Work out the finished part from the listing and answer in its coordinate system (mm). Face numbers are marked on the shaded views. Coordinates: 2 decimals unless noted, no trailing zeros. Loops run counter-clockwise (first coordinate to the right, second up) from the corner with the lowest first, then second, coordinate; pieces in that order, holes last. Notation, with made-up numbers: (53, -29) - (94, -29) arc R36 ccw to (94, 6) - close; hole circle Ø7 at (89, 2.5). An arc over 180 degrees is marked (long way). Write each question's results on one line, items separated by ' | '. Start each with the question number.
Item 1: For a pull along X with two mould halves and no side action, classify the marked faces 1 and 2 as +X half, -X half, draft (parallel to the pull), parting line (faces both ways), or undercut.
Item 2: Section B-B, the plane z = -7 is taken. Write down the section's boundary in (x, y).
Item 3: Section A-A, the plane x = -4 is taken. Write down the section's boundary in (y, z).
Item 4: Section D-D, the plane y = 4.5 is taken. Count the separate pieces of the cut face and the enclosed holes in it, plus the area to 3 significant figures.
Item 5: Section C-C, the plane z = 32.06 is taken. Write down the section's boundary in (x, y) (3 decimals), plus the area to 3 significant figures.
Item 6: Consider probe 1 along X at (y, z) = (5.15, -35) (3 decimals); probe 2 along X at (y, z) = (2.3, -21.4) (3 decimals); probe 3 along Z at (x, y) = (17.5, 5). Determine where each line is inside the solid, lowest interval first. Write a range as [from, to].
Item 7: Each of these flat-tipped pins is pushed along its axis until it touches: pin 1 Ø1 at (y, z) = (1, -3) entering from +X; pin 2 Ø10 at (x, z) = (-19.75, 32.06) entering from -Y; pin 3 Ø1.8 at (x, z) = (22.5, -6) entering from +Y; pin 4 Ø3 at (x, z) = (-19.5, 31) entering from +Y. Where does it stop, or does it pass through?
from build123d import *

# Parameters (mm, degrees)
SKETCH1_W           = 50.8
SKETCH1_H           = 50.8
SKETCH1_R           = 1.375
SKETCH1_W_2         = 40.8
SKETCH1_H_2         = 40.8
BOSS_EXTRUDE1_DEPTH = 1.5
SKETCH2_W           = 50.8
SKETCH2_H           = 50.8
SKETCH2_W_2         = 47.8
SKETCH2_H_2         = 47.8
BOSS_EXTRUDE2_DEPTH = 5
FILLET2_R           = 3
BOSS_EXTRUDE3_REACH = 38.504
SKETCH5_R           = 5
SKETCH5_R_2         = 1.375
SKETCH6_R           = 2.55
CUT_EXTRUDE1_DEPTH  = 3
SKETCH7_R           = 1.55
BOSS_EXTRUDE4_DEPTH = 6.5
SKETCH8_R           = 3.125
CUT_EXTRUDE2_DEPTH  = 4
FILLET3_R           = 5
BOSS_EXTRUDE5_DEPTH = 6.5
SKETCH10_R          = 3.125
CUT_EXTRUDE3_DEPTH  = 4
SKETCH11_R          = 1.55
CUT_EXTRUDE4_DEPTH  = 50.27727671
FILLET4_R           = 3


with BuildPart() as part:
    # Sketch1 → Boss-Extrude1 (new body)
    with BuildSketch(Plane(origin=(0, 0, 0), x_dir=(1, 0, 0), z_dir=(0, 1, 0))):
        Rectangle(SKETCH1_W, SKETCH1_H)
        with Locations(Location((-21.4, 21.4, 0), (0, 0, 270))):
            Circle(SKETCH1_R, mode=Mode.SUBTRACT)
        with Locations(Location((21.4, 21.4, 0), (0, 0, 270))):
            Circle(SKETCH1_R, mode=Mode.SUBTRACT)
        with Locations(Location((21.4, -21.4, 0), (0, 0, 270))):
            Circle(SKETCH1_R, mode=Mode.SUBTRACT)
        with Locations(Location((-21.4, -21.4, 0), (0, 0, 270))):
            Circle(SKETCH1_R, mode=Mode.SUBTRACT)
        Rectangle(SKETCH1_W_2, SKETCH1_H_2, mode=Mode.SUBTRACT)
    extrude(amount=BOSS_EXTRUDE1_DEPTH)

    # Sketch2 → Boss-Extrude2 (add)
    with BuildSketch(Plane(origin=(0, 1.5, 0), x_dir=(1, 0, 0), z_dir=(0, 1, 0))):
        Rectangle(SKETCH2_W, SKETCH2_H)
        Rectangle(SKETCH2_W_2, SKETCH2_H_2, mode=Mode.SUBTRACT)
    extrude(amount=BOSS_EXTRUDE2_DEPTH)

    # Fillet2
    fillet2_edges = [part.edges().sort_by_distance(p)[0] for p in [
        (23.9, 4, -23.9),
        (-23.9, 4, -23.9),
        (-23.9, 4, 23.9),
        (23.9, 4, 23.9),
        (25.4, 3.25, 25.4),
        (-25.4, 3.25, 25.4),
        (-25.4, 3.25, -25.4),
        (25.4, 3.25, -25.4),
    ]]
    fillet(fillet2_edges, radius=FILLET2_R)

    # Boss-Extrude3: up to this face of the body (flat: up to its plane)
    boss_extrude3_end = Plane(part.part.faces().sort_by_distance((0, 0, -24.68157951))[0])
    # Sketch5 → Boss-Extrude3 (add, up to the picked face)
    with BuildSketch(Plane(origin=(0, 6.5, 0), x_dir=(1, 0, 0), z_dir=(0, 1, 0)), mode=Mode.PRIVATE) as boss_extrude3_sk1:
        with Locations((-21.4, 21.4)):
            Circle(SKETCH5_R)
        with Locations(Location((-21.4, 21.4, 0), (0, 0, 270))):
            Circle(SKETCH5_R_2, mode=Mode.SUBTRACT)
    boss_extrude3_tool1 = split(extrude(boss_extrude3_sk1.sketch, amount=-BOSS_EXTRUDE3_REACH, mode=Mode.PRIVATE), bisect_by=boss_extrude3_end, keep=Keep.BOTH, mode=Mode.PRIVATE)
    # Sketch5 → Boss-Extrude3 (add, up to the picked face)
    with BuildSketch(Plane(origin=(0, 6.5, 0), x_dir=(1, 0, 0), z_dir=(0, 1, 0)), mode=Mode.PRIVATE) as boss_extrude3_sk2:
        with Locations((21.4, 21.4)):
            Circle(SKETCH5_R)
        with Locations(Location((21.4, 21.4, 0), (0, 0, 270))):
            Circle(SKETCH5_R_2, mode=Mode.SUBTRACT)
    boss_extrude3_tool2 = split(extrude(boss_extrude3_sk2.sketch, amount=-BOSS_EXTRUDE3_REACH, mode=Mode.PRIVATE), bisect_by=boss_extrude3_end, keep=Keep.BOTH, mode=Mode.PRIVATE)
    # Sketch5 → Boss-Extrude3 (add, up to the picked face)
    with BuildSketch(Plane(origin=(0, 6.5, 0), x_dir=(1, 0, 0), z_dir=(0, 1, 0)), mode=Mode.PRIVATE) as boss_extrude3_sk3:
        with Locations((21.4, -21.4)):
            Circle(SKETCH5_R)
        with Locations(Location((21.4, -21.4, 0), (0, 0, 270))):
            Circle(SKETCH5_R_2, mode=Mode.SUBTRACT)
    boss_extrude3_tool3 = split(extrude(boss_extrude3_sk3.sketch, amount=-BOSS_EXTRUDE3_REACH, mode=Mode.PRIVATE), bisect_by=boss_extrude3_end, keep=Keep.BOTH, mode=Mode.PRIVATE)
    # Sketch5 → Boss-Extrude3 (add, up to the picked face)
    with BuildSketch(Plane(origin=(0, 6.5, 0), x_dir=(1, 0, 0), z_dir=(0, 1, 0)), mode=Mode.PRIVATE) as boss_extrude3_sk4:
        with Locations((-21.4, -21.4)):
            Circle(SKETCH5_R)
        with Locations(Location((-21.4, -21.4, 0), (0, 0, 270))):
            Circle(SKETCH5_R_2, mode=Mode.SUBTRACT)
    boss_extrude3_tool4 = split(extrude(boss_extrude3_sk4.sketch, amount=-BOSS_EXTRUDE3_REACH, mode=Mode.PRIVATE), bisect_by=boss_extrude3_end, keep=Keep.BOTH, mode=Mode.PRIVATE)
    add(boss_extrude3_tool1.solids().sort_by(Axis((-26.258579, 6.5, -21.4), (0, -1, 0)))[0])
    add(boss_extrude3_tool2.solids().sort_by(Axis((16.541421, 6.5, -21.4), (0, -1, 0)))[0])
    add(boss_extrude3_tool3.solids().sort_by(Axis((16.541421, 6.5, 21.4), (0, -1, 0)))[0])
    add(boss_extrude3_tool4.solids().sort_by(Axis((-26.258579, 6.5, 21.4), (0, -1, 0)))[0])

    # Sketch6 → Cut-Extrude1 (cut)
    with BuildSketch(Plane(origin=(0, 6.5, 0), x_dir=(1, 0, 0), z_dir=(0, 1, 0))):
        with Locations(Location((-21.4, 21.4, 0), (0, 0, 270))):
            Circle(SKETCH6_R)
        with Locations(Location((21.4, 21.4, 0), (0, 0, 270))):
            Circle(SKETCH6_R)
        with Locations(Location((-21.4, -21.4, 0), (0, 0, 270))):
            Circle(SKETCH6_R)
        with Locations(Location((21.4, -21.4, 0), (0, 0, 270))):
            Circle(SKETCH6_R)
    extrude(amount=-CUT_EXTRUDE1_DEPTH, mode=Mode.SUBTRACT)

    # Sketch7 → Boss-Extrude4 (add)
    with BuildSketch(Plane(origin=(0, 6.5, 0), x_dir=(1, 0, 0), z_dir=(0, 1, 0))):
        with BuildLine():
            Line((16.5, 25.4), (16.5, 40))
            Line((16.5, 40), (28.5, 40))
            Line((28.5, 40), (28.5, 32.25))
            Line((28.5, 32.25), (25.4, 24.4))
            ThreePointArc((25.4, 24.4), (22.107106781, 26.349747468), (18.4, 25.4))
            Line((18.4, 25.4), (16.5, 25.4))
        make_face()
        with Locations(Location((22.5, 35, 0), (0, 0, 270))):
            Circle(SKETCH7_R, mode=Mode.SUBTRACT)
    boss_extrude4 = extrude(amount=-BOSS_EXTRUDE4_DEPTH)

    # Sketch8 → Cut-Extrude2 (cut)
    with BuildSketch(Plane(origin=(0, 6.5, 0), x_dir=(1, 0, 0), z_dir=(0, 1, 0))):
        with Locations(Location((22.5, 35, 0), (0, 0, 270))):
            Circle(SKETCH8_R)
    cut_extrude2 = extrude(amount=-CUT_EXTRUDE2_DEPTH, mode=Mode.SUBTRACT)

    # Mirror1: Boss-Extrude4, Cut-Extrude2 across plane
    add(boss_extrude4.mirror(Plane(origin=(0, 0, 0), x_dir=(0, 0, 1), z_dir=(1, 0, 0))))
    add(cut_extrude2.mirror(Plane(origin=(0, 0, 0), x_dir=(0, 0, 1), z_dir=(1, 0, 0))), mode=Mode.SUBTRACT)

    # Fillet3
    fillet3_edges = [part.edges().sort_by_distance(p)[0] for p in [
        (16.5, 3.25, -25.4),
        (-16.5, 3.25, -25.4),
    ]]
    fillet(fillet3_edges, radius=FILLET3_R)

    # Sketch9 → Boss-Extrude5 (add)
    with BuildSketch(Plane(origin=(0, 6.5, 0), x_dir=(1, 0, 0), z_dir=(0, 1, 0))):
        with BuildLine():
            Line((-24.25, -25.50822346), (-24.25, -36.962430679))
            ThreePointArc((-24.25, -36.962430679), (-19.755484827, -37.480943602), (-15.25, -37.893410284))
            Line((-15.25, -37.893410284), (-15.25, -25.4))
            Line((-15.25, -25.4), (-18.4, -25.4))
            ThreePointArc((-18.4, -25.4), (-21.30751714, -26.399144619), (-24.25, -25.50822346))
        make_face()
    boss_extrude5 = extrude(amount=-BOSS_EXTRUDE5_DEPTH)

    # Sketch10 → Cut-Extrude3 (cut)
    with BuildSketch(Plane(origin=(0, 6.5, 0), x_dir=(1, 0, 0), z_dir=(0, 1, 0))):
        with Locations(Location((-19.75, -32.06, 0), (0, 0, 270))):
            Circle(SKETCH10_R)
    cut_extrude3 = extrude(amount=-CUT_EXTRUDE3_DEPTH, mode=Mode.SUBTRACT)

    # Sketch11 → Cut-Extrude4 (cut, through all)
    with BuildSketch(Plane(origin=(0, 2.5, 0), x_dir=(1, 0, 0), z_dir=(0, 1, 0))):
        with Locations(Location((-19.75, -32.06, 0), (0, 0, 270))):
            Circle(SKETCH11_R)
    cut_extrude4 = extrude(amount=-CUT_EXTRUDE4_DEPTH, mode=Mode.SUBTRACT)

    # Mirror2: Boss-Extrude5, Cut-Extrude3, Cut-Extrude4 across plane
    add(boss_extrude5.mirror(Plane(origin=(0, 0, 0), x_dir=(0, 0, 1), z_dir=(1, 0, 0))))
    add(cut_extrude3.mirror(Plane(origin=(0, 0, 0), x_dir=(0, 0, 1), z_dir=(1, 0, 0))), mode=Mode.SUBTRACT)
    add(cut_extrude4.mirror(Plane(origin=(0, 0, 0), x_dir=(0, 0, 1), z_dir=(1, 0, 0))), mode=Mode.SUBTRACT)

    # Fillet4
    fillet4_edges = [part.edges().sort_by_distance(p)[0] for p in [
        (-24.25, 3.25, 25.50822346),
        (-15.25, 3.25, 25.4),
        (15.25, 3.25, 25.4),
        (24.25, 3.25, 25.50822346),
    ]]
    fillet(fillet4_edges, radius=FILLET4_R)


solid = part.part
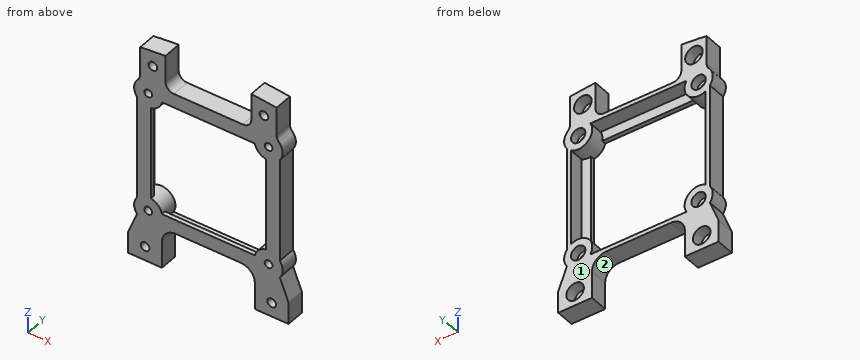
Answer key:
1) face 1: draft | face 2: undercut
2) outline: (-25.4, 0) - (-20.4, 0) - (-20.4, 1.5) - (-23.9, 1.5) - (-23.9, 6.5) - (-25.4, 6.5) - close; (20.4, 0) - (25.4, 0) - (25.4, 6.5) - (23.9, 6.5) - (23.9, 1.5) - (20.4, 1.5) - close
3) outline: (0, -25.4) - (6.5, -25.4) - (6.5, -23.9) - (1.5, -23.9) - (1.5, -20.4) - (0, -20.4) - close; (0, 20.4) - (1.5, 20.4) - (1.5, 23.9) - (6.5, 23.9) - (6.5, 25.4) - (0, 25.4) - close
4) separate pieces: 1 | enclosed holes: 9 | area: 870 mm^2
5) outline: (-24.25, 0) - (-21.3, 0) - (-21.3, 2.5) - (-22.875, 2.5) - (-22.875, 6.5) - (-24.25, 6.5) - close; (-18.2, 0) - (-15.25, 0) - (-15.25, 6.5) - (-16.625, 6.5) - (-16.625, 2.5) - (-18.2, 2.5) - close; (15.25, 0) - (18.2, 0) - (18.2, 2.5) - (16.625, 2.5) - (16.625, 6.5) - (15.25, 6.5) - close; (21.3, 0) - (24.25, 0) - (24.25, 6.5) - (22.875, 6.5) - (22.875, 2.5) - (21.3, 2.5) - close | area: 51.5 mm^2
6) probe 1: x = [-28.5, -25.625], [-19.375, -16.5], [16.5, 19.375], [25.625, 28.5] | probe 2: x = [-26.4, -22.775], [-20.025, -16.4], [16.4, 20.025], [22.775, 26.4] | probe 3: z = [-40, -18.27], [18.27, 29.89], [34.23, 37.7]
7) pin 1: stops at x = 25.4 | pin 2: stops at y = 0 | pin 3: stops at y = 1.5 | pin 4: stops at y = 2.5
